For this review, take the finished solid that the model builds, in its own axes (mm). Face numbers are marked on the shaded views. Coordinates: 2 decimals unless noted, no trailing zeros. Order: outer loops, then holes, each group sorted by start corner. A loop starts at its lowest first (then second) coordinate and runs counter-clockwise, first axis right, second up.
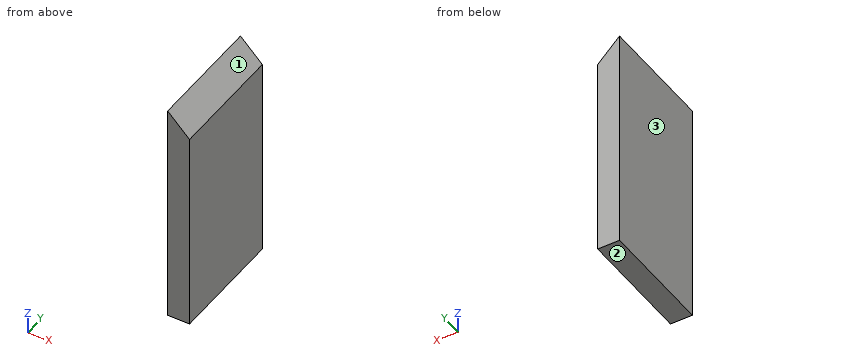
from build123d import *

# Parameters (mm, degrees)
F0_W     = 101.6
F0_H     = 196.85
F1_DEPTH = 19.05
F2_SIZE  = 19.04999


# Not quite as in the source:
# - a fillet or chamfer is up to 0.001 mm smaller than in the source, because OpenCascade refuses the exact size


with BuildPart() as f1:
    # F0 (on Right) → F1 (new body)
    with BuildSketch(Plane.YZ):
        with Locations((-6.1650511805, 0)):
            Rectangle(F0_W, F0_H)
    extrude(amount=F1_DEPTH)

    # F2 (size 19.05 in the source; OpenCascade refuses exactly that, so slightly less here)
    f2_edges = [f1.edges().sort_by_distance(p)[0] for p in [
        (19.05, -6.165051, 98.425),
    ]]
    chamfer(f2_edges, length=F2_SIZE)


solid = f1.part
1. To check wall thickness, follow L1, parallel to Z at x = 15.5, y = 2.5 (3 decimals); L2, parallel to Z at x = 2.75, y = -3 (3 decimals); L3, parallel to X at y = 28.5, z = 88. State the ranges of each line that lie inside material, in increasing order.
Answer below:
L1: z = -98.425 to 82.925
L2: z = -98.425 to 95.675
L3: x = 0 to 10.43
2. Clearance check with a flat-ended pin moving along its axis: pin 1 Ø4 at (y, z) = (-42, -40) entering from -X. State where the tip first meets the part, or that it passes through.
Answer below:
pin 1: stops at x = 0
3. The part is to be moulded in two halves that separate along X. For the marked faces 1, 2 and 3, say which applies: +X half, -X half, draft (parallel to the pull), parting line (faces both ways), or undercut.
Answer below:
face 1: +X half
face 2: draft
face 3: -X half
4. Take a section at B-B, the plane x = 7.75. Give the boundary of the cut face in (y, z) (3 decimals).
Answer below:
outline: (-56.965, -98.425) - (44.635, -98.425) - (44.635, 90.675) - (-56.965, 90.675) - close
